Part model, mm, in its own coordinate system. Coordinates: 2 decimals unless noted, no trailing zeros. Loops run counter-clockwise (first coordinate to the right, second up) from the corner with the lowest first, then second, coordinate; pieces in that order, holes last. Notation, with made-up numbers: (67, 11) - (74, 11) arc R13 ccw to (74, 25) - close; hole circle Ø6 at (31.5, -19). An arc over 180 degrees is marked (long way). Use a Markdown table: item, result. Add a question column.
1) Band-saw the part on A-A (z = 1.4). Give the number of separate pieces and of enclosed holes in the cut face, plus the area to 3 significant figures.
2) Probe probe 1 along Y at (x, z) = (-0.5, 3.4); probe 2 along Y at (x, z) = (-0.75, 0.7); probe 3 along X at (y, z) = (17.5, 2.95). List the from-to ranges inside material, lowest first. Write a range as [from, to].
3) Band-saw the part on C-C (x = 1). Give the cut face in (y, z), plus the area to 3 significant figures.
4) Band-saw the part on D-D (x = -2.5). Give the cut face in (y, z).
5) Band-saw the part on B-B (y = 20). Give the cut face in (x, z), plus the area to 3 significant figures.
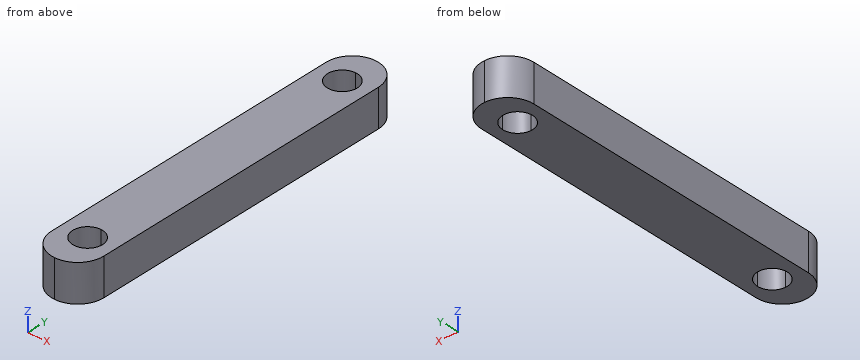
from build123d import *

# Parameters (mm, degrees)
BOSS_EXTRUDE1_DEPTH = 5
FILLET1_R           = 3.5


with BuildPart() as part:
    # Sketch1 → Boss-Extrude1 (new body)
    with BuildSketch(Plane.XY):
        with BuildLine():
            Line((0, -21.32), (0, -24.32))
            Line((0, -24.32), (3.5, -24.32))
            Line((3.5, -24.32), (3.5, 24.32))
            Line((3.5, 24.32), (0, 24.32))
            Line((0, 24.32), (0, 21.32))
            ThreePointArc((0, 21.32), (1.414213562, 20.734213562), (2, 19.32))
            ThreePointArc((2, 19.32), (1.414213562, 17.905786438), (0, 17.32))
            Line((0, 17.32), (0, -17.32))
            ThreePointArc((0, -17.32), (1.414213562, -17.905786438), (2, -19.32))
            ThreePointArc((2, -19.32), (1.414213562, -20.734213562), (0, -21.32))
        make_face()
        with BuildLine():
            Line((-3.5, -24.32), (0, -24.32))
            Line((0, -24.32), (0, -21.32))
            ThreePointArc((0, -21.32), (-2, -19.32), (0, -17.32))
            Line((0, -17.32), (0, 17.32))
            ThreePointArc((0, 17.32), (-2, 19.32), (0, 21.32))
            Line((0, 21.32), (0, 24.32))
            Line((0, 24.32), (-3.5, 24.32))
            Line((-3.5, 24.32), (-3.5, -24.32))
        make_face()
    extrude(amount=BOSS_EXTRUDE1_DEPTH)

    # Fillet1
    fillet1_edges = [part.edges().sort_by_distance(p)[0] for p in [
        (-3.5, 24.32, 2.5),
        (3.5, 24.32, 2.5),
        (-3.5, -24.32, 2.5),
        (3.5, -24.32, 2.5),
    ]]
    fillet(fillet1_edges, radius=FILLET1_R - 0.0001)  # a hair under: the kernel refuses the full size


solid = part.part
Answer block:
| question | item | result |
|---|---|---|
| 1 | separate pieces | 1 |
| 1 | enclosed holes | 2 |
| 1 | area | 305 mm2 |
| 2 | probe 1 | [-24.28, -21.26], [-17.38, 17.38], [21.26, 24.28] |
| 2 | probe 2 | [-24.24, -21.17], [-17.47, 17.47], [21.17, 24.24] |
| 2 | probe 3 | [-3.5, -0.83], [0.83, 3.5] |
| 3 | outline | (-24.17, 0) - (-21.05, 0) - (-21.05, 5) - (-24.17, 5) - close; (-17.59, 0) - (17.59, 0) - (17.59, 5) - (-17.59, 5) - close; (21.05, 0) - (24.17, 0) - (24.17, 5) - (21.05, 5) - close |
| 3 | area | 207 mm2 |
| 4 | outline | (-23.27, 0) - (23.27, 0) - (23.27, 5) - (-23.27, 5) - close |
| 5 | outline | (-3.5, 0) - (-1.88, 0) - (-1.88, 5) - (-3.5, 5) - close; (1.88, 0) - (3.5, 0) - (3.5, 5) - (1.88, 5) - close |
| 5 | area | 16.2 mm2 |
